The figure shows three views and two pictorial views of one solid part (mm, origin at its lowest corner). Answer the questions. A direction names the side the tool comes from. Round coordinates to 2 decimals unless told otherwise and drop trailing zeros. Order: outer loops, then holes, each group sorted by start corner. A loop starts at its lowest first (then second) coordinate and runs counter-clockwise, first axis right, second up. Notation, with made-up numbers: (-33, 81) -> (23, 81) arc R25 cw to (23, 105) -> close; hole circle Ø6 at (-28, 4). An arc over 180 degrees is marked (long way). Return JSON: item names as keys, results as strings. Group by question number.
(1) The part is cut by section D-D (z = 14). Determine the outline of the cut face in (x, y).
(2) Determine the mould class of the marked faces 4, 5 and 6 for opening direction Z: +Z half, -Z half, draft (parallel to the pull), parting line (faces both ways), or undercut.
(3) The part is cut by section C-C (y = 31). Determine the outline of the cut face in (x, z).
(4) The part is cut by section B-B (z = 11). Determine the outline of the cut face in (x, y) (1 decimal).
(5) Consider line 1 (Y direction, x = 28, z = 13.75); line 2 (Z direction, x = 31, y = 35); line 3 (Y direction, x = 24.5, z = 12). Determine where each line is inside the solid, lowest interval first. Write a range as [from, to].
(6) Each of these flat-tipped pins is pushed along its axis until it touches: pin 1 (3 mm diameter, centred on x = 20.5, y = 7, fed in from +Z); pin 2 (4 mm diameter, centred on x = 22.5, z = 12.5, fed in from -Y); pin 3 (1 mm diameter, centred on x = 17, z = 10.5, fed in from +Y). Where does it stop, or does it pass through?
(7) Which of the six approach directions +Z, -Z, +X, -X, +Y, -Y give full straight-line access (tool end or side, diameter ignored) to the marked faces 1, 2 and 3?
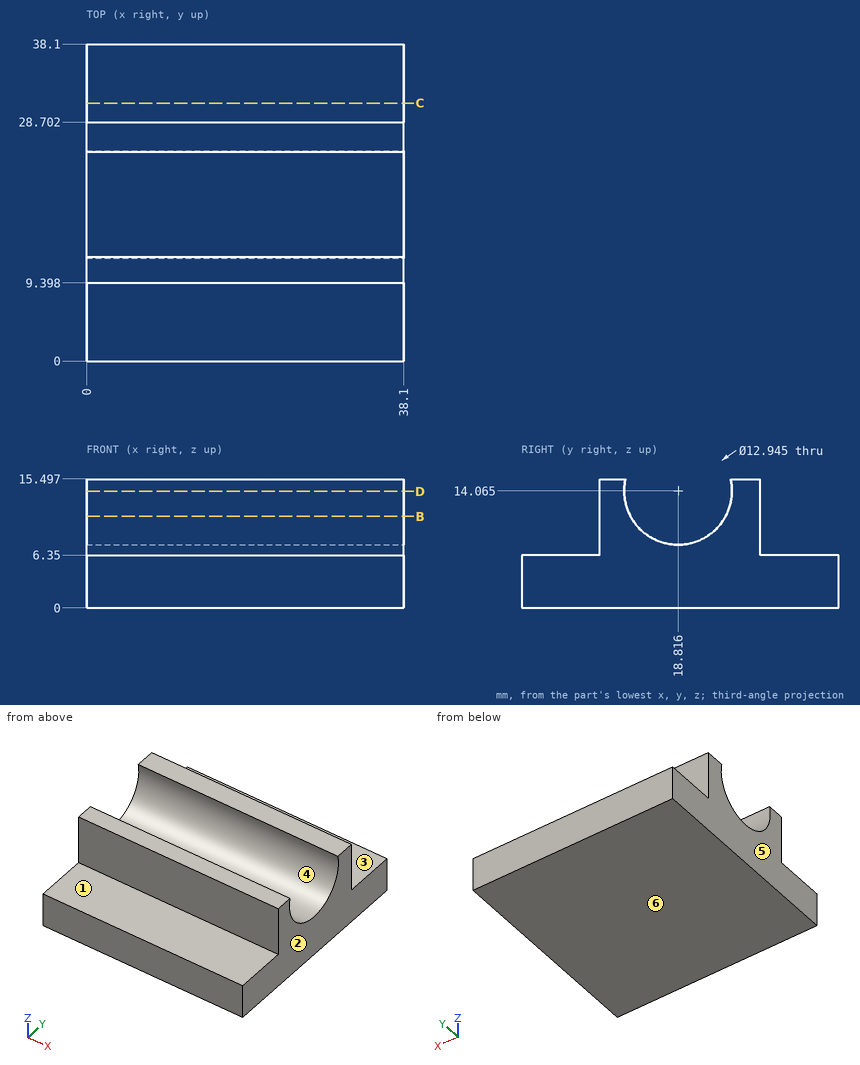
Answer below:
{
 "1": {"outline": "(0, 9.4) -> (38.1, 9.4) -> (38.1, 12.34) -> (0, 12.34) -> close; (0, 25.29) -> (38.1, 25.29) -> (38.1, 28.7) -> (0, 28.7) -> close"},
 "2": {"face 4": "undercut", "face 5": "draft", "face 6": "-Z half"},
 "3": {"outline": "(0, 0) -> (38.1, 0) -> (38.1, 6.35) -> (0, 6.35) -> close"},
 "4": {"outline": "(0, 9.4) -> (38.1, 9.4) -> (38.1, 13.1) -> (0, 13.1) -> close; (0, 24.5) -> (38.1, 24.5) -> (38.1, 28.7) -> (0, 28.7) -> close"},
 "5": {"line 1": "y = [9.4, 12.35], [25.28, 28.7]", "line 2": "z = [0, 6.35]", "line 3": "y = [9.4, 12.68], [24.95, 28.7]"},
 "6": {"pin 1": "stops at z = 6.35", "pin 2": "stops at y = 9.4", "pin 3": "stops at y = 28.7"},
 "7": {"face 1": "+Z, +X, -X, -Y", "face 2": "+Z, -Z, +X, +Y, -Y", "face 3": "+Z, +X, -X, +Y"}
}
